from build123d import *

# Parameters (mm, degrees)
SKETCH1_R           = 2.6
BOSS_EXTRUDE1_DEPTH = 1.6
SKETCH2_R           = 2
BOSS_EXTRUDE2_DEPTH = 2.4
SKETCH3_R           = 2.35
BOSS_EXTRUDE3_DEPTH = 1
CHAMFER1_SIZE       = 0.75
CHAMFER1_SIZE2      = 0.832959386
FILLET1_R           = 0.2
SCALE1_SCALE        = 1.15


with BuildPart() as part:
    # Sketch1 → Boss-Extrude1 (new body)
    with BuildSketch(Plane(origin=(0, 0, 0), x_dir=(1, 0, 0), z_dir=(0, 1, 0))):
        Circle(SKETCH1_R)
    extrude(amount=BOSS_EXTRUDE1_DEPTH)

    # Sketch2 → Boss-Extrude2 (add)
    with BuildSketch(Plane(origin=(0, 1.6, 0), x_dir=(1, 0, 0), z_dir=(0, 1, 0))):
        Circle(SKETCH2_R)
    extrude(amount=BOSS_EXTRUDE2_DEPTH)

    # Sketch3 → Boss-Extrude3 (add)
    with BuildSketch(Plane(origin=(0, 4, 0), x_dir=(1, 0, 0), z_dir=(0, 1, 0))):
        Circle(SKETCH3_R)
    extrude(amount=BOSS_EXTRUDE3_DEPTH)

    # Chamfer1
    chamfer1_edges = [part.edges().sort_by_distance(p)[0] for p in [
        (-2.35, 5, 0),
    ]]
    chamfer1_side = [part.faces().sort_by_distance(p)[0] for p in [
        (-2.35, 4.5, 0),
    ]]
    chamfer(chamfer1_edges, length=CHAMFER1_SIZE, length2=CHAMFER1_SIZE2, reference=chamfer1_side[0])

    # Fillet1
    fillet1_edges = [part.edges().sort_by_distance(p)[0] for p in [
        (-1.517040614, 5, 0),
        (-2.35, 4.25, 0),
        (-2, 1.6, 0),
    ]]
    fillet(fillet1_edges, radius=FILLET1_R)


with BuildPart() as part_1:
    # Scale1: scaled about (-4.4e-08, 2.199734094, 0)
    add(part.part.scale(SCALE1_SCALE).moved(Location((7e-09, -0.329960114, 0))))


solid = part_1.part
Could you check a few things on this model? Use its own coordinates, in mm. Coordinates: 2 decimals unless noted, no trailing zeros. Write each loop counter-clockwise with the first axis right and the second up, starting at its lowest first coordinate (ties: lowest second). Pieces come first, ordered by that corner, then holes. Notation, with made-up numbers: (6, 8) - (53, 8) arc R24 cw to (53, 21) - close; hole circle Ø3 at (16.5, 3.25). An arc over 180 degrees is marked (long way). Put each result on its own line as item: value. Start each with the question number.
Q1. I want a section at A-A on y = 3.4. Write out the boundary of the cut face in (x, z), plus the area to 3 significant figures.
Q2. Thinking about a two-plate mould opening in Y: for faces 1 (the cylindrical face through (-2.298, 2.987, -0.101)), 2 (the flat face through (0, 5.42, 0)), 3 (the flat face through (0, -0.33, 0)), which applies, pulls with the +Y half, pulls with the -Y half, needs draft (parallel to the pull), parting line crosses it, or undercut?
Q3. I'm going to push flat-ended pins straight in: P1, Ø2, axis at y = 1.5, z = 1.5, coming from the +X side; P2, Ø3, axis at x = 0, y = 4.5, coming from the -Z side. Where does each tip first touch, or does it pass through?
Q4. I want a section at B-B on y = 4.9. Write out the boundary of the cut face in (x, z), plus the area to 3 significant figures.
Q5. Please list where these lines run through material, in increasing order: L1, parallel to Z at x = -0.45, y = 4.6; L2, parallel to Z at x = 1.6, y = 0.1; L3, parallel to X at y = 1.7, z = -0.55.
Checks:
1. outline: circle Ø4.6 at (0, 0)
1. area: 16.6 mm²
2. face 1: undercut
2. face 2: pulls with the +Y half
2. face 3: pulls with the -Y half
3. P1: x = 2.95
3. P2: z = -2.7
4. outline: circle Ø4.64 at (0, 0)
4. area: 16.9 mm²
5. L1: -2.61 to 2.61
5. L2: -2.53 to 2.53
5. L3: -2.24 to 2.24
